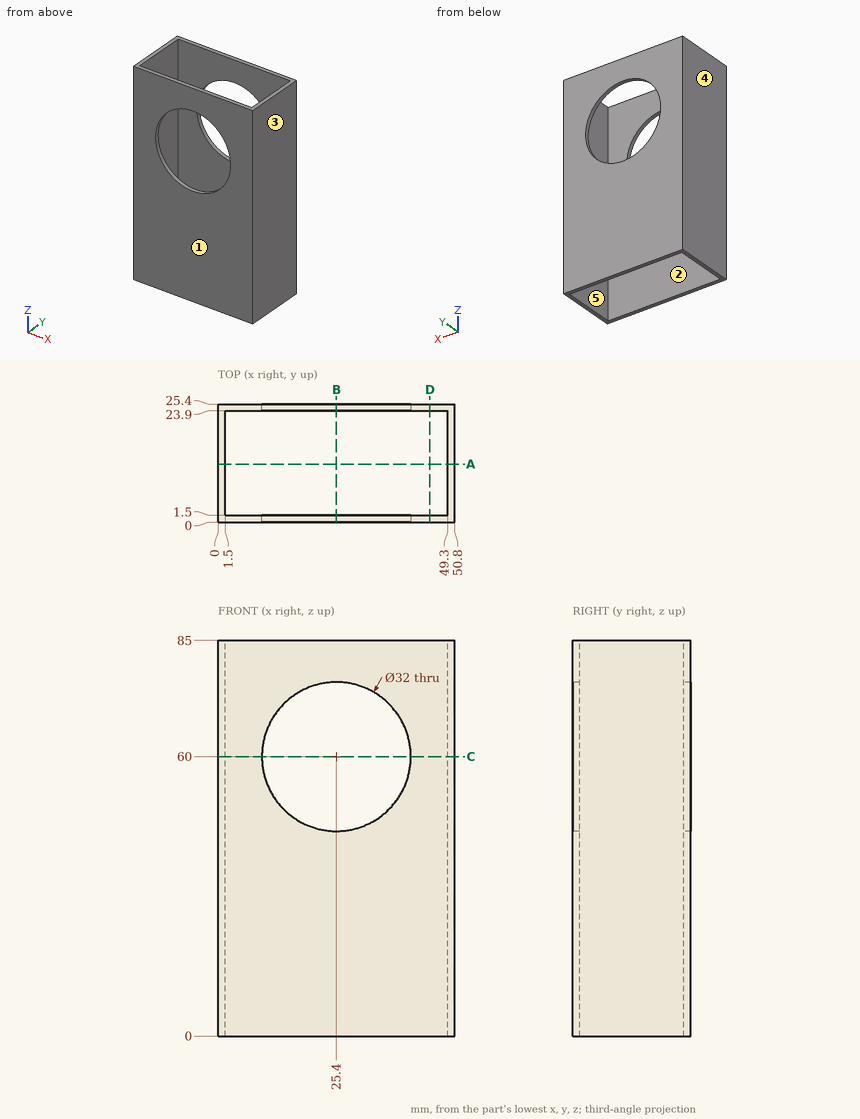
The figure shows three views and two pictorial views of one solid part (mm, origin at its lowest corner). Answer the questions. A direction names the side the tool comes from. Give positions to 0.01 mm unless a question says otherwise; leave off trailing zeros. Loops run counter-clockwise (first coordinate to the right, second up) from the corner with the lowest first, then second, coordinate; pieces in that order, holes last. Notation, with made-up numbers: (31.5, 59) -> (70.5, 59) arc R14 cw to (70.5, 65) -> close; hole circle Ø2 at (3, 40). An arc over 180 degrees is marked (long way). Use a Markdown table: item, result. Add a question column.
1. Find the intervals of material crossed by probe 1 along X at (y, z) = (13.5, 72); probe 2 along Z at (x, y) = (25.4, 24.65); probe 3 along X at (y, z) = (1, 60), in increasing order.
2. Section B-B on x = 25.4 is taken. Determine the outline of the cut face in (y, z), and give its area (3 significant figures).
3. For the marked faces 1 and 2, determine the directions among +Z, -Z, +X, -X, +Y, -Y from which every point of the face is accessible in a straight line to the end or side of a thin tool.
4. Section D-D on x = 45.5 is taken. Determine the outline of the cut face in (y, z).
5. Determine the mould class of the marked faces 3, 4 and 5 for opening direction X: released by +X, released by -X, zero draft, split by the parting line, or undercut.
6. Section A-A on y = 12.5 is taken. Determine the outline of the cut face in (x, z), and give its area (3 significant figures).
7. Section C-C on z = 60 is taken. Determine the outline of the cut face in (x, y).
Results below:
| question | item | result |
|---|---|---|
| 1 | probe 1 | x = 0 to 1.5, 49.3 to 50.8 |
| 1 | probe 2 | z = 0 to 44, 76 to 85 |
| 1 | probe 3 | x = 0 to 9.4, 41.4 to 50.8 |
| 2 | outline | (0, 0) -> (1.5, 0) -> (1.5, 44) -> (0, 44) -> close; (0, 76) -> (1.5, 76) -> (1.5, 85) -> (0, 85) -> close; (23.9, 0) -> (25.4, 0) -> (25.4, 44) -> (23.9, 44) -> close; (23.9, 76) -> (25.4, 76) -> (25.4, 85) -> (23.9, 85) -> close |
| 2 | area | 159 mm^2 |
| 3 | face 1 | +Z, -Z, +X, -X, -Y |
| 3 | face 2 | +Z, -Z |
| 4 | outline | (0, 0) -> (1.5, 0) -> (1.5, 85) -> (0, 85) -> close; (23.9, 0) -> (25.4, 0) -> (25.4, 85) -> (23.9, 85) -> close |
| 5 | face 3 | released by +X |
| 5 | face 4 | released by -X |
| 5 | face 5 | undercut |
| 6 | outline | (0, 0) -> (1.5, 0) -> (1.5, 85) -> (0, 85) -> close; (49.3, 0) -> (50.8, 0) -> (50.8, 85) -> (49.3, 85) -> close |
| 6 | area | 255 mm^2 |
| 7 | outline | (0, 0) -> (9.4, 0) -> (9.4, 1.5) -> (1.5, 1.5) -> (1.5, 23.9) -> (9.4, 23.9) -> (9.4, 25.4) -> (0, 25.4) -> close; (41.4, 0) -> (50.8, 0) -> (50.8, 25.4) -> (41.4, 25.4) -> (41.4, 23.9) -> (49.3, 23.9) -> (49.3, 1.5) -> (41.4, 1.5) -> close |
